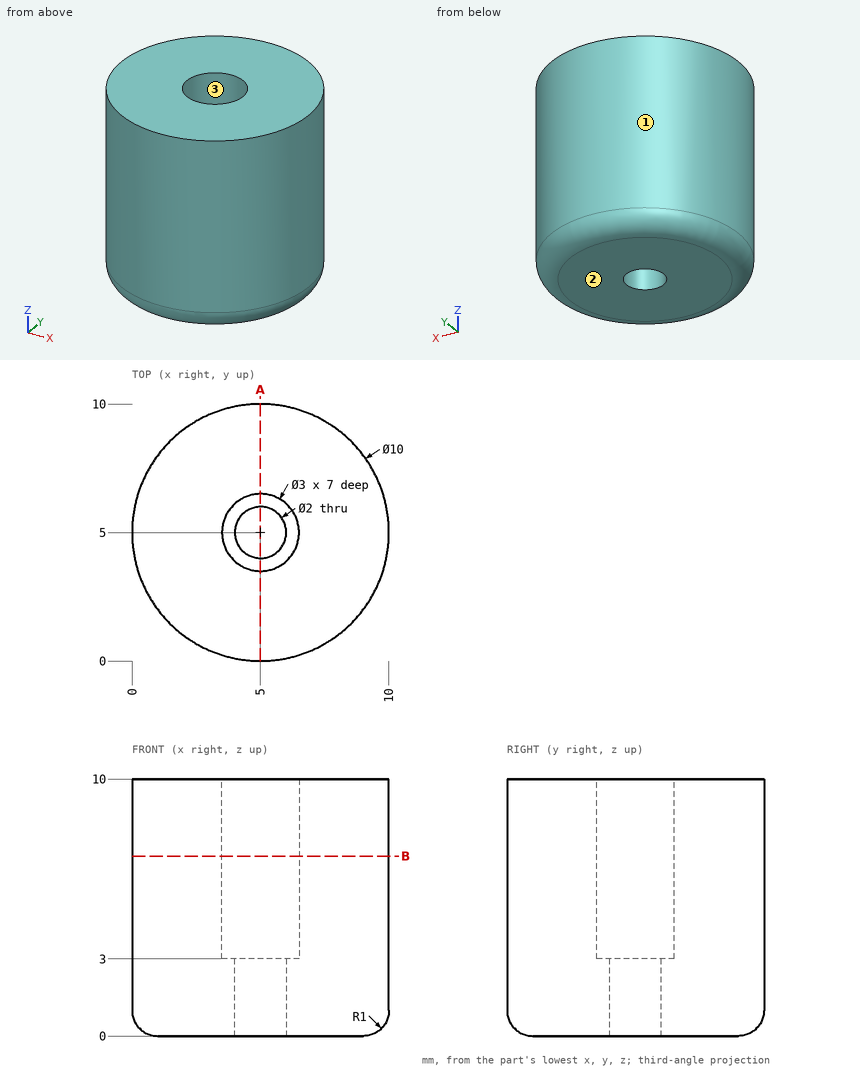
The drawing under review shows one solid part. Ordinate dimensions are in mm from its lowest x, y, z. Round coordinates to 2 decimals unless told otherwise and drop trailing zeros. Loops run counter-clockwise (first coordinate to the right, second up) from the corner with the lowest first, then second, coordinate; pieces in that order, holes last. Notation, with made-up numbers: (44.25, 73) - (74.25, 73) arc R33 cw to (74.25, 103) - close; hole circle Ø2 at (34, 57). An arc over 180 degrees is marked (long way). Use a Markdown table: item, result. Add a question column.
Q1. Add section A-A (x = 5). State the section outline as (y, z) points.
Q2. For probe 1 along Y at (x, z) = (5, 5); probe 2 along Y at (x, z) = (5.5, 6.5); probe 3 along X at (y, z) = (2, 7.25), list the stretches that pass through material, from the lowest coordinate up.
Q3. Insertion check: pin 1 Ø1.5 at (x, y) = (5, 5.5) entering from +Z; pin 2 Ø1.8 at (x, y) = (5, 5) entering from -Z. Each pin has a flat end and moves straight along its axis. Give the tip position at first contact, or say it passes through.
Q4. The part is to be moulded in two halves that separate along Y. For the marked faces 1, 2 and 3, say which applies: pulls with the +Y half, pulls with the -Y half, needs draft (parallel to the pull), parting line crosses it, or undercut.
Q5. Add section B-B (z = 7). State the section outline as (x, y) points.
Worked answers:
| question | item | result |
|---|---|---|
| 1 | outline | (0, 1) arc R1 ccw to (1, 0) - (4, 0) - (4, 3) - (3.5, 3) - (3.5, 10) - (0, 10) - close; (6, 0) - (9, 0) arc R1 ccw to (10, 1) - (10, 10) - (6.5, 10) - (6.5, 3) - (6, 3) - close |
| 2 | probe 1 | 0 to 3.5, 6.5 to 10 |
| 2 | probe 2 | 0.03 to 3.59, 6.41 to 9.97 |
| 2 | probe 3 | 1 to 9 |
| 3 | pin 1 | z = 3 |
| 3 | pin 2 | through |
| 4 | face 1 | parting line crosses it |
| 4 | face 2 | needs draft |
| 4 | face 3 | undercut |
| 5 | outline | circle Ø10 at (5, 5); hole circle Ø3 at (5, 5) |
